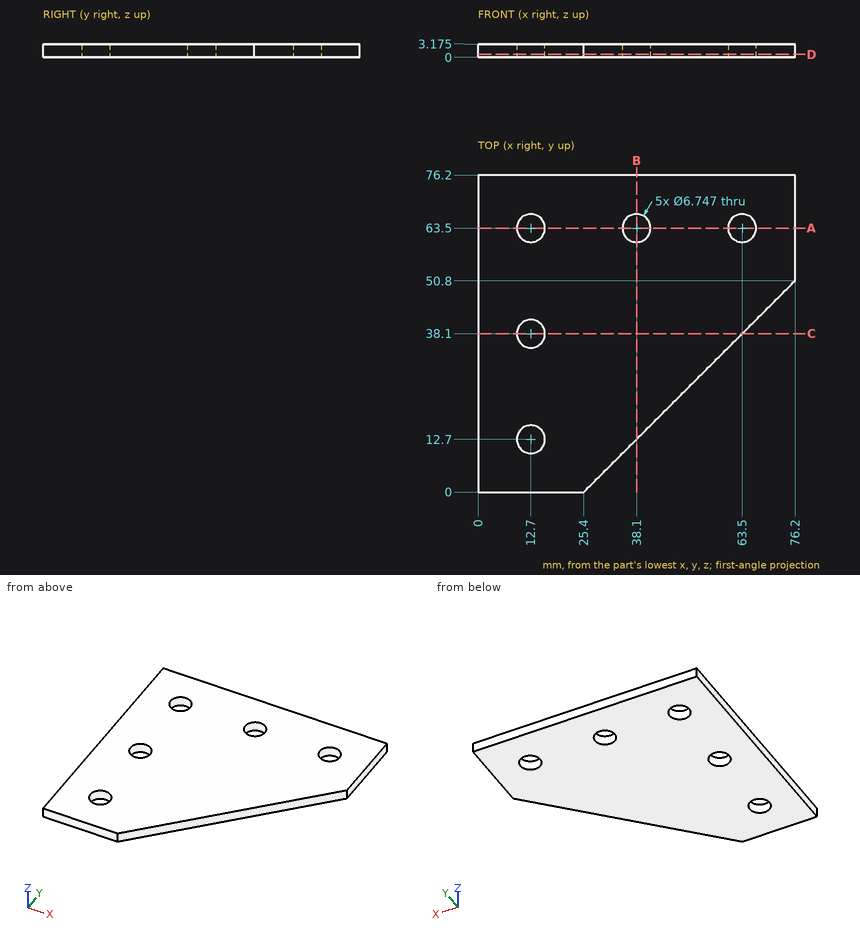
Part print with two shaded views. Sizes in mm from the minimum x, y, z corner. Round coordinates to 2 decimals unless told otherwise and drop trailing zeros. Order: outer loops, then holes, each group sorted by start corner. A loop starts at its lowest first (then second) coordinate and runs counter-clockwise, first axis right, second up. Notation, with made-up numbers: (-12, -26.75) - (8, -26.75) arc R15 ccw to (8, -9.75) - close; hole circle Ø6 at (-4, 19.25). An arc over 180 degrees is marked (long way). Answer as CSV lines item,"result". Start each with the question number.
1. Saw through at B-B, the plane x = 38.1. Write the cut outline in (y, z) (1 decimal).
2. Drill centre lines: L1, parallel to Y at x = 12.7, z = 1.1; L2, parallel to X at y = 61, z = 1 (1 decimal); L3, parallel to X at y = 64.5, z = 0.1. Where is each one in solid material? Low to high. Write a range as [from, to].
3. Saw through at C-C, the plane y = 38.1. Write the cut outline in (x, z) (1 decimal).
4. Saw through at D-D, the plane z = 0.7. Write the cut outline in (x, y).
5. Saw through at A-A, the plane y = 63.5. Write the cut outline in (x, z) (1 decimal), and give its area (3 significant figures).
Model answer:
1,outline,"(12.7, 0) - (60.1, 0) - (60.1, 3.2) - (12.7, 3.2) - close; (66.9, 0) - (76.2, 0) - (76.2, 3.2) - (66.9, 3.2) - close"
2,L1,"y = [0, 9.33], [16.07, 34.73], [41.47, 60.13], [66.87, 76.2]"
2,L2,"x = [0, 10.4], [15, 35.8], [40.4, 61.2], [65.8, 76.2]"
2,L3,"x = [0, 9.48], [15.92, 34.88], [41.32, 60.28], [66.72, 76.2]"
3,outline,"(0, 0) - (9.3, 0) - (9.3, 3.2) - (0, 3.2) - close; (16.1, 0) - (63.5, 0) - (63.5, 3.2) - (16.1, 3.2) - close"
4,outline,"(0, 0) - (25.4, 0) - (76.2, 50.8) - (76.2, 76.2) - (0, 76.2) - close; hole circle Ø6.75 at (12.7, 12.7); hole circle Ø6.75 at (12.7, 38.1); hole circle Ø6.75 at (12.7, 63.5); hole circle Ø6.75 at (38.1, 63.5); hole circle Ø6.75 at (63.5, 63.5)"
5,outline,"(0, 0) - (9.3, 0) - (9.3, 3.2) - (0, 3.2) - close; (16.1, 0) - (34.7, 0) - (34.7, 3.2) - (16.1, 3.2) - close; (41.5, 0) - (60.1, 0) - (60.1, 3.2) - (41.5, 3.2) - close; (66.9, 0) - (76.2, 0) - (76.2, 3.2) - (66.9, 3.2) - close"
5,area,"178 mm²"
